from build123d import *

# Parameters (mm, degrees)
SKETCH10_W          = 50.8
SKETCH10_H          = 50.8
BOSS_EXTRUDE4_DEPTH = 50.8
CUT_EXTRUDE6_DEPTH  = 77.2
SKETCH19_W          = 44.45
SKETCH19_H          = 44.45
CUT_EXTRUDE8_DEPTH  = 47.625
BOSS_EXTRUDE6_DEPTH = 47.625


with BuildPart() as part:
    # Sketch10 → Boss-Extrude4 (new body)
    with BuildSketch(Plane(origin=(0, 0, 0), x_dir=(1, 0, 0), z_dir=(0, 1, 0))):
        Rectangle(SKETCH10_W, SKETCH10_H)
    extrude(amount=BOSS_EXTRUDE4_DEPTH)

    # Sketch17 → Cut-Extrude6 (cut, through all)
    with BuildSketch(Plane.XY.offset(25.4)):
        Polygon((25.4, 0), (25.4, 50.8), (11.788181024, 0), align=None)
    extrude(amount=-CUT_EXTRUDE6_DEPTH, mode=Mode.SUBTRACT)

    # Sketch19 → Cut-Extrude8 (cut)
    with BuildSketch(Plane(origin=(0, 50.8, 0), x_dir=(1, 0, 0), z_dir=(0, 1, 0))):
        Rectangle(SKETCH19_W, SKETCH19_H)
    extrude(amount=-CUT_EXTRUDE8_DEPTH, mode=Mode.SUBTRACT)

    # Sketch20 → Boss-Extrude6 (add)
    with BuildSketch(Plane.XY.offset(25.4)):
        Polygon((22.225, 50.8), (8.613181024, 0), (11.788181024, 0), (25.4, 50.8), align=None)
    extrude(amount=-BOSS_EXTRUDE6_DEPTH)


solid = part.part
The listing builds one solid part. Answer for the finished solid, in the listing's coordinates (mm). A direction names the side the tool comes from. Coordinates: 2 decimals unless noted, no trailing zeros. Loops run counter-clockwise (first coordinate to the right, second up) from the corner with the lowest first, then second, coordinate; pieces in that order, holes last. Notation, with made-up numbers: (-1.5, -19.75) -> (11.5, -19.75) arc R13 cw to (11.5, -8.75) -> close; hole circle Ø3 at (48, -30.5). An arc over 180 degrees is marked (long way). Answer in a Markdown table with one row per item. Add a question column.
1. Determine the mould class of faces 1 (the flat face through (-5, 27, 22.225)), 2 (the flat face through (-6, 25, -25.4)), 3 (the flat face through (18.7, 25.8, 0.4)) for opening direction X: +X half, -X half, draft (parallel to the pull), parting line (faces both ways), or undercut.
2. The part is cut by section C-C, the plane z = 4.5. Write down the section's boundary in (x, y) (3 decimals).
3. The part is cut by section D-D, the plane y = 6.5. Write down the section's boundary in (x, z) (3 decimals), then the cut area to 3 significant figures.
4. The part is cut by section A-A, the plane y = 21.5. Write down the section's boundary in (x, z) (3 decimals).
5. For faces 4 (the flat face through (15.934, 27.321, 0.311)), 5 (the flat face through (-6, 25, 25.4)), determine the directions among +Z, -Z, +X, -X, +Y, -Y from which every point of the face is accessible in a straight line to the end or side of a thin tool.
6. A flat-ended cylindrical pin translates along its axis: P1, Ø13.5, axis at y = 27.5, z = -1, coming from the +X side. Find the tip coordinate at first contact, or state that the pin passes through.
7. Consider line 1 (Z direction, x = -1.5, y = 11) (3 decimals); line 2 (Y direction, x = 0, z = 13.5) (3 decimals); line 3 (X direction, y = 26, z = -4) (3 decimals). Determine where each line is inside the solid, lowest interval first. Write a range as [from, to].
8. The part is cut by section B-B, the plane x = -19. Write down the section's boundary in (y, z) (3 decimals).
Answer below:
| question | item | result |
|---|---|---|
| 1 | face 1 | undercut |
| 1 | face 2 | draft |
| 1 | face 3 | +X half |
| 2 | outline | (-25.4, 0) -> (11.788, 0) -> (25.4, 50.8) -> (22.225, 50.8) -> (9.464, 3.175) -> (-22.225, 3.175) -> (-22.225, 50.8) -> (-25.4, 50.8) -> close |
| 3 | outline | (-25.4, -25.4) -> (13.53, -25.4) -> (13.53, 25.4) -> (-25.4, 25.4) -> close; hole (-22.225, -22.225) -> (10.355, -22.225) -> (10.355, 22.225) -> (-22.225, 22.225) -> close |
| 3 | area | 529 mm2 |
| 4 | outline | (-25.4, -25.4) -> (17.549, -25.4) -> (17.549, 25.4) -> (-25.4, 25.4) -> close; hole (-22.225, -22.225) -> (14.374, -22.225) -> (14.374, 22.225) -> (-22.225, 22.225) -> close |
| 5 | face 4 | +Y |
| 5 | face 5 | +Z, +X, -X, +Y, -Y |
| 6 | P1 | x = 20.97 |
| 7 | line 1 | [-25.4, -22.225], [22.225, 25.4] |
| 7 | line 2 | [0, 3.175] |
| 7 | line 3 | [-25.4, -22.225], [15.58, 18.755] |
| 8 | outline | (0, -25.4) -> (50.8, -25.4) -> (50.8, -22.225) -> (3.175, -22.225) -> (3.175, 22.225) -> (50.8, 22.225) -> (50.8, 25.4) -> (0, 25.4) -> close |
